Input: part model. Units: mm. Frame: model coordinates. Coordinates: 2 decimals unless noted, no trailing zeros. Order: outer loops, then holes, each group sorted by start corner. A loop starts at its lowest first (then second) coordinate and runs counter-clockwise, first axis right, second up.
from build123d import *

# Parameters (mm, degrees)
F0_R     = 25.4
F1_DEPTH = 1.524


with BuildPart() as f1:
    # F0 (on Front) → F1 (new body)
    with BuildSketch(Plane.XZ):
        Circle(F0_R)
        with BuildLine():
            Line((-10.722334, 7.286357), (-10.722334, 15.24))
            Line((-10.722334, 15.24), (-9.452334, 15.24))
            Line((-9.452334, 15.24), (-9.456435, 7.166546))
            ThreePointArc((-9.456435, 7.166546), (-12.20241, 3.061331), (-17.045993, 4.027183))
            Line((-17.045993, 4.027183), (-16.151985, 4.920356))
            ThreePointArc((-16.151985, 4.920356), (-12.630592, 4.252393), (-10.722334, 7.286357))
        make_face(mode=Mode.SUBTRACT)
        Polygon((-4.88111, 2.723804), (-8.317264, 15.24), (-7.000273, 15.24), (-4.163434, 4.906811), (-1.746424, 14.153804), (-0.977187, 14.153804), (1.561451, 4.906811), (4.262375, 15.24), (5.575043, 15.24), (2.303517, 2.723804), (0.843776, 2.723804), (-1.341137, 10.682351), (-3.421369, 2.723804), align=None, mode=Mode.SUBTRACT)
    extrude(amount=F1_DEPTH)


solid = f1.part
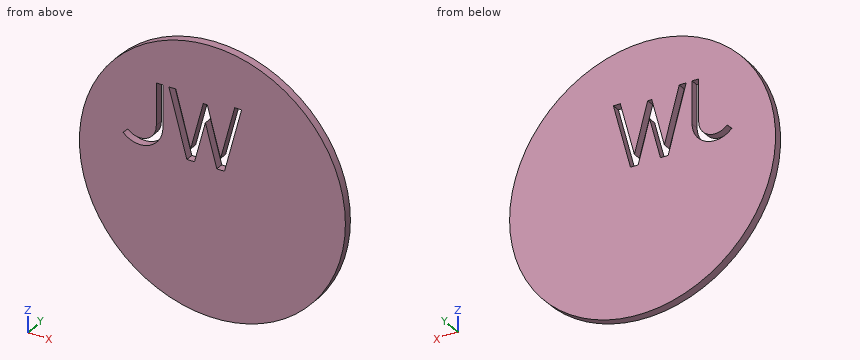
Item 1: Cut plane A-A on y = -0.35. Return loops of the section in (x, z) (3 decimals).
Response values:
outline: circle Ø50.8 at (0, 0); hole (-17.046, 4.027) arc R4.445 ccw to (-9.456, 7.167) - (-9.452, 15.24) - (-10.722, 15.24) - (-10.722, 7.286) arc R3.181 cw to (-16.152, 4.92) - close; hole (-8.317, 15.24) - (-4.881, 2.724) - (-3.421, 2.724) - (-1.341, 10.682) - (0.844, 2.724) - (2.304, 2.724) - (5.575, 15.24) - (4.262, 15.24) - (1.561, 4.907) - (-0.977, 14.154) - (-1.746, 14.154) - (-4.163, 4.907) - (-7, 15.24) - close
Item 2: Ray query, probe 1 along X at (y, z) = (-0.85, 12.5); probe 2 along X at (y, z) = (-0.2, 7); probe 3 along Z at (x, y) = (-14, -0.3). Return the intervals inside material, ascending.
Response values:
probe 1: x = -22.11 to -10.72, -9.45 to -7.57, -6.25 to -2.18, -0.52 to 3.55, 4.86 to 22.11
probe 2: x = -24.42 to -10.72, -9.46 to -6.06, -4.74 to -3.62, -2.3 to -0.33, 0.99 to 2.11, 3.42 to 24.42
probe 3: z = -21.19 to 2.72, 3.99 to 21.19
Item 3: Cut plane C-C on x = -14. Return loops of the section in (y, z), then the cut area to 3 significant figures.
Response values:
outline: (-1.52, -21.19) - (0, -21.19) - (0, 2.72) - (-1.52, 2.72) - close; (-1.52, 3.99) - (0, 3.99) - (0, 21.19) - (-1.52, 21.19) - close
area: 62.7 mm2
Item 4: Cut plane B-B on x = 0. Return loops of the section in (y, z), then the cut area to 3 significant figures.
Response values:
outline: (-1.52, -25.4) - (0, -25.4) - (0, 5.8) - (-1.52, 5.8) - close; (-1.52, 10.59) - (0, 10.59) - (0, 25.4) - (-1.52, 25.4) - close
area: 70.1 mm2
Item 5: Cut plane D-D on z = -17. Return loops of the section in (x, y).
Response values:
outline: (-18.87, -1.52) - (18.87, -1.52) - (18.87, 0) - (-18.87, 0) - close
Item 6: Pin query (flat end, axial travel): pin 1 Ø0.8 at (x, y) = (-1.5, -1) entering from -Z. Return the tip coordinate at first contact, or that it passes through.
Response values:
pin 1: stops at z = -25.38
